from build123d import *

# Parameters (mm, degrees)
SKETCH1_W           = 29
SKETCH1_H           = 12.7
BOSS_EXTRUDE1_DEPTH = 15.7
SKETCH2_R           = 0.65
BOSS_EXTRUDE2_DEPTH = 3.7
FILLET1_R           = 1


with BuildPart() as part:
    # Sketch1 → Boss-Extrude1 (new body)
    with BuildSketch(Plane(origin=(0, 0, 0), x_dir=(1, 0, 0), z_dir=(0, 1, 0))):
        Rectangle(SKETCH1_W, SKETCH1_H)
    extrude(amount=BOSS_EXTRUDE1_DEPTH)

    # Sketch2 → Boss-Extrude2 (add)
    with BuildSketch(Plane(origin=(0, 15.7, 0), x_dir=(1, 0, 0), z_dir=(0, 1, 0))):
        with Locations(Location((12.5, -3.8, 0), (0, 0, 90))):
            Circle(SKETCH2_R)
        with Locations(Location((-12.5, -3.8, 0), (0, 0, 90))):
            Circle(SKETCH2_R)
        with Locations(Location((-7.5, 3.2, 0), (0, 0, 90))):
            Circle(SKETCH2_R)
        with Locations(Location((-2.5, -3.8, 0), (0, 0, 90))):
            Circle(SKETCH2_R)
        with Locations(Location((12.5, 3.7, 0), (0, 0, 90))):
            Circle(SKETCH2_R)
        with Locations(Location((-2.5, 3.2, 0), (0, 0, 90))):
            Circle(SKETCH2_R)
        with Locations(Location((-7.5, -3.8, 0), (0, 0, 90))):
            Circle(SKETCH2_R)
        with Locations(Location((-12.5, 3.2, 0), (0, 0, 90))):
            Circle(SKETCH2_R)
    extrude(amount=BOSS_EXTRUDE2_DEPTH)

    # Fillet1
    fillet1_edges = [part.edges().sort_by_distance(p)[0] for p in [
        (0, 0, 6.35),
        (-14.5, 0, 0),
        (0, 0, -6.35),
        (14.5, 0, 0),
    ]]
    fillet(fillet1_edges, radius=FILLET1_R)


solid = part.part
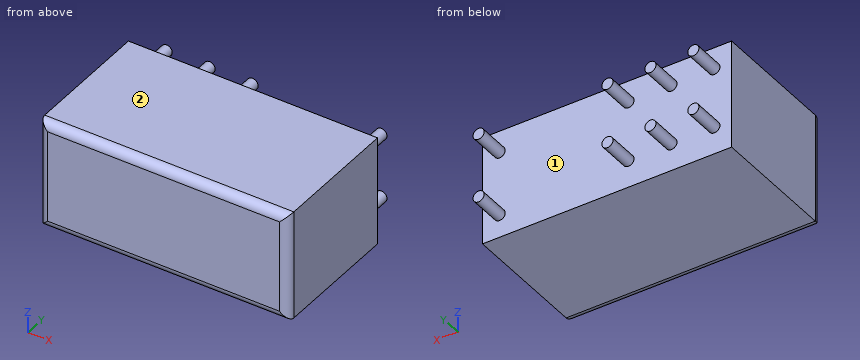
For this review, take the finished solid that the model builds, in its own axes (mm). Face numbers are marked on the shaded views. A direction names the side the tool comes from. Round coordinates to 2 decimals unless told otherwise and drop trailing zeros. Order: outer loops, then holes, each group sorted by start corner. A loop starts at its lowest first (then second) coordinate and runs counter-clockwise, first axis right, second up. Notation, with made-up numbers: M 58.25,82 L 64.25,82 A26 ccw 64.25,113 Z; hole C 88.5,14.5 d2. An arc over 180 degrees is marked long. Use a Markdown table: item, result. Add a question column.
Item 1: Add section C-C, the plane x = -7.5. Give the boundary of the cut face in (y, z), then the cut area to 3 significant figures.
Item 2: Add section A-A, the plane y = 16. Give the boundary of the cut face in (x, z), then the cut area to 3 significant figures.
Item 3: To check wall thickness, follow line 1 along Y through (x, z) = (-7.5, 4.5). State the ranges of the line that lie inside material, in increasing order.
Item 4: Add section D-D, the plane x = -4.25. Give the boundary of the cut face in (y, z), then the cut area to 3 significant figures.
Item 5: Insertion check: pin 1 (1 mm diameter, centred on x = -11.5, z = -5, fed in from +Y). The pin has a flat end and moves straight along its axis. Give the tip position at first contact, or say it passes through.
Item 6: Tool access review of the marked faces 1 and 2: name each direction out of +Z, -Z, +X, -X, +Y, -Y from which nothing blocks a thin tool from reaching the whole face with its end or side.
Item 7: Add section B-B, the plane z = 3.8. Give the boundary of the cut face in (x, y), then the cut area to 3 significant figures.
Geometry results:
| question | item | result |
|---|---|---|
| 1 | outline | M 0,-5.35 A1 ccw 1,-6.35 L 15.7,-6.35 L 15.7,-3.85 L 19.4,-3.85 L 19.4,-2.55 L 15.7,-2.55 L 15.7,3.15 L 19.4,3.15 L 19.4,4.45 L 15.7,4.45 L 15.7,6.35 L 1,6.35 A1 ccw 0,5.35 Z |
| 1 | area | 209 mm² |
| 2 | outline | C -12.5,-3.2 d1.3; C -12.5,3.8 d1.3; C -7.5,-3.2 d1.3; C -7.5,3.8 d1.3; C -2.5,-3.2 d1.3; C -2.5,3.8 d1.3; C 12.5,-3.7 d1.3; C 12.5,3.8 d1.3 |
| 2 | area | 10.6 mm² |
| 3 | line 1 | y = 0 to 15.7 |
| 4 | outline | M 0,-5.35 A1 ccw 1,-6.35 L 15.7,-6.35 L 15.7,6.35 L 1,6.35 A1 ccw 0,5.35 Z |
| 4 | area | 199 mm² |
| 5 | pin 1 | stops at y = 15.7 |
| 6 | face 1 | +Y |
| 6 | face 2 | +Z, +X, -X, +Y, -Y |
| 7 | outline | M -14.5,1 A1 ccw -13.5,0 L 13.5,0 A1 ccw 14.5,1 L 14.5,15.7 L 13.15,15.7 L 13.15,19.4 L 11.85,19.4 L 11.85,15.7 L -1.85,15.7 L -1.85,19.4 L -3.15,19.4 L -3.15,15.7 L -6.85,15.7 L -6.85,19.4 L -8.15,19.4 L -8.15,15.7 L -11.85,15.7 L -11.85,19.4 L -13.15,19.4 L -13.15,15.7 L -14.5,15.7 Z |
| 7 | area | 474 mm² |
